Autodesk Inventor part; units mm, degrees
ref_plane "YZ Plane" through (0, 0, 0) normal (1, 0, 0) x (0, 1, 0)
ref_plane "XZ Plane" through (0, 0, 0) normal (0, 1, 0) x (-1, 0, 0)
ref_plane "XY Plane" through (0, 0, 0) normal (0, 0, 1) x (1, 0, 0)
sketch "Sketch1" plane through (0, 0, 0) normal (0, 1, 0) x (-1, 0, 0)
  line L0 (0, 0) -> (88.9, 0)
  line L1 (88.9, 0) -> (88.9, 70.104)
  line L2 (88.9, 70.104) -> (0, 70.104)
  line L3 (0, 70.104) -> (0, 0)
  dimension "d6" = 88.9
  dimension "d7" = 70.104
extrude "Extrusion1" add sketch "Sketch1" along normal blind 3.175
sketch "Sketch2" plane through (0, 0, 0) normal (0, -1, 0) x (1, 0, 0)
  line L0 (0, 0) -> (-88.9, 0)
  line L1 (0, 70.104) -> (0, 0)
  line L2 (-88.9, 70.104) -> (0, 70.104)
  line L3 (-88.9, 0) -> (-88.9, 70.104)
  circle A0 centre (-44.45, 35.052) radius 6.35
  dimension "d8" = 12.7
  dimension "d9" = 44.45
  dimension "d10" = 44.45
  dimension "d11" = 35.052
  dimension "d12" = 35.052
extrude "Extrusion2" cut sketch "Sketch2" against normal through all contours A0
equation "\"d9\" = d10"
equation "\"d11\" = d12"
properties part number "zMotorMount"
Read the model definition and answer for the solid it produces. Units are mm, in the model's axes. Round coordinates to 2 decimals unless told otherwise and drop trailing zeros. Write each loop counter-clockwise with the first axis right and the second up, starting at its lowest first coordinate (ties: lowest second). Pieces come first, ordered by that corner, then holes. Notation, with made-up numbers: M -17.75,-2 L -6.75,-2 A24 cw -6.75,13 Z; hole C 79.25,16.5 d7. An arc over 180 degrees is marked long. Use a Markdown table: item, result.
1) The part is cut by section A-A (x = -44.45). Write down the section's boundary in (y, z) (3 decimals).
Answers follow:
| item | result |
|---|---|
| outline | M 0,0 L 3.175,0 L 3.175,28.702 L 0,28.702 Z; M 0,41.402 L 3.175,41.402 L 3.175,70.104 L 0,70.104 Z |
2) A straight line is drawn through the part: line 1 along Z through (x, y) = (-44.45, 0.7). Find the intervals that lie inside material, in ascending order. Write a range as [from, to].
Answers follow:
| item | result |
|---|---|
| line 1 | z = [0, 28.7], [41.4, 70.1] |
3) For a pull along Z with two mould halves and no side action, classify faces 1 (the flat face through (-44, 2, 0)), 2 (the flat face through (-45, 2, 70.104)), 3 (the flat face through (-44, 0, 43)), 4 (the cylindrical face through (-38.584, 1.565, 32.62)) as pulls with the +Z half, pulls with the -Z half, needs draft (parallel to the pull), parting line crosses it, or undercut.
Answers follow:
| item | result |
|---|---|
| face 1 | pulls with the -Z half |
| face 2 | pulls with the +Z half |
| face 3 | needs draft |
| face 4 | undercut |
4) The part is cut by section C-C (y = 0.8). Write down the section's boundary in (x, z), plus the area to 3 significant figures.
Answers follow:
| item | result |
|---|---|
| outline | M -88.9,0 L 0,0 L 0,70.1 L -88.9,70.1 Z; hole C -44.45,35.05 d12.7 |
| area | 6,110 mm2 |
5) The part is cut by section B-B (z = 33). Write down the section's boundary in (x, y) (3 decimals).
Answers follow:
| item | result |
|---|---|
| outline | M -88.9,0 L -50.459,0 L -50.459,3.175 L -88.9,3.175 Z; M -38.441,0 L 0,0 L 0,3.175 L -38.441,3.175 Z |
